Work out the finished part from the listing and answer in its coordinate system (mm). Coordinates: 2 decimals unless noted, no trailing zeros. Order: outer loops, then holes, each group sorted by start corner. A loop starts at its lowest first (then second) coordinate and runs counter-clockwise, first axis right, second up. Notation, with made-up numbers: M 4,-37.75 L 48,-37.75 A15 cw 48,-18.75 Z; hole C 64.5,-8 d3. An arc over 180 degrees is marked long. Use a Markdown table: item, result.
Solid Edge part; units mm, degrees
sketch "Sketch1" plane through (0, 0, 0) normal (0, 0, 1) x (1, 0, 0)
  line L0 (-2, 0) -> (-2, 1.55)
  line L1 (-2, 1.55) -> (-1.8, 1.75)
  line L2 (-1.8, 1.75) -> (0, 1.75)
  line L3 (0, 1.75) -> (0, 1)
  line L4 (0, 1) -> (9.7545, 1)
  line L5 (9.7545, 1) -> (10, 0.7545)
  line L6 (10, 0.7545) -> (10, 0)
  line L7 (10, 0) -> (-2, 0)
revolve "RevolvedProtrusion1" add sketch "Sketch1" angle 360 about axis through (10, 0, 0) along (-1, 0, 0)
cosmetic_thread "Thread1"
sketch "Sketch2" plane through (-2, 0, 0) normal (1, 0, 0) x (0, 1, 0)
  line L0 (-0.433, 0.75) -> (-0.866, 0)
  line L1 (-0.866, 0) -> (-0.433, -0.75)
  line L2 (-0.433, -0.75) -> (0.433, -0.75)
  line L3 (0.433, -0.75) -> (0.866, 0)
  line L4 (0.866, 0) -> (0.433, 0.75)
  line L5 (0.433, 0.75) -> (-0.433, 0.75)
extrude "ExtrudedCutout_1" cut sketch "Sketch2" along normal blind 1
hole "Hole_1" at (-1, 0, 0) direction (1, 0, 0) diameter 0.8 depth 11 countersink diameter 1.7321 countersink angle 120
properties part number "SVSS-M2-10"
(1) A cutting plane is placed at A-A (y = 0). Determine the outline of the cut face in (x, z).
Conclusion:
| item | result |
|---|---|
| outline | M -2,-1.55 L -1.8,-1.75 L 0,-1.75 L 0,-1 L 9.75,-1 L 10,-0.75 L 10,-0.4 L -0.73,-0.4 L -1,-0.87 L -1,-0.75 L -2,-0.75 Z; M -2,0.75 L -1,0.75 L -1,0.87 L -0.73,0.4 L 10,0.4 L 10,0.75 L 9.75,1 L 0,1 L 0,1.75 L -1.8,1.75 L -2,1.55 Z |
(2) Given P1, Ø1.5, axis at x = 2, y = 1, coming from the -Z side; P2, Ø1.5, axis at x = 7.5, z = -1, coming from the -Y side; P3, Ø1.5, axis at x = 2, y = 0, coming from the +Z side, each flat-ended and moving along its own axis, determine where each tip first touches the part or whether it passes through.
Conclusion:
| item | result |
|---|---|
| P1 | z = -0.97 |
| P2 | y = -0.97 |
| P3 | z = 1 |
(3) A cutting plane is placed at B-B (x = 0.25). Determine the outline of the cut face in (y, z), then the cut area to 3 significant figures.
Conclusion:
| item | result |
|---|---|
| outline | C 0,0 d2; hole C 0,0 d0.8 |
| area | 2.64 mm2 |
(4) Determine the mould class of faces 1 (the flat face through (-1.5, 0, -0.75)), 2 (the cylindrical face through (5, 0, -1)), 3 (the flat face through (-1.5, 0, 0.75)), 4 (the flat face through (0, 1, 1)) for opening direction Z: pulls with the +Z half, pulls with the -Z half, needs draft (parallel to the pull), parting line crosses it, or undercut.
Conclusion:
| item | result |
|---|---|
| face 1 | undercut |
| face 2 | parting line crosses it |
| face 3 | undercut |
| face 4 | needs draft |
(5) Straight lines are drawn through the part: L1, parallel to Y at x = 5.75, z = 0; L2, parallel to X at y = 1, z = 0.75. For each, find the intervals that lie inside material, in ascending order.
Conclusion:
| item | result |
|---|---|
| L1 | -1 to -0.4, 0.4 to 1 |
| L2 | -2 to 0 |
